Source: CAD feature listing. Evaluate the final solid. Frame: model axes, mm. A direction names the side the tool comes from. Coordinates: 2 decimals unless noted, no trailing zeros. Loops run counter-clockwise (first coordinate to the right, second up) from the corner with the lowest first, then second, coordinate; pieces in that order, holes last. Notation, with made-up numbers: (31.5, 72.5) - (66.5, 72.5) arc R19 ccw to (66.5, 94.5) - close; hole circle Ø4 at (66, -31). An arc over 180 degrees is marked (long way). Use CSV: the item, a comma, the result in double quotes. Start each with the question number.
```python
from build123d import *

# Parameters (mm, degrees)
FASE1_SIZE                      = 2
FASE2_SIZE                      = 4
FASE2_SIZE2                     = 1.377310453
FASE3_SIZE                      = 4
FASE3_SIZE2                     = 1.377310453
SCHNITT_LINEAR_AUSTRAGEN1_DEPTH = 9.5
FASE4_SIZE                      = 1
FASE4_SIZE2                     = 1.613032213
FASE5_SIZE                      = 1.623645291


with BuildPart() as part:
    # Skizze1 → Rotation1 (revolve)
    with BuildSketch(Plane.XY, mode=Mode.PRIVATE) as rotation1_sk:
        with BuildLine():
            Line((-2.51871264, 34.081541744), (-2.51871264, 15.53217569))
            Line((-2.51871264, 15.53217569), (-5.248906592, 12.857142857))
            ThreePointArc((-5.248906592, 12.857142857), (-7.478321416, 8.069832253), (-6, 3))
            Line((-6, 3), (-10, 3))
            Line((-10, 3), (-10, 15))
            Line((-10, 15), (-6, 15))
            Line((-6, 15), (-4.093652292, 16.867831662))
            Line((-4.093652292, 16.867831662), (-4.093652292, 20.696496392))
            ThreePointArc((-4.093652292, 20.696496392), (-7.464630082, 27.878319169), (-2.51871264, 34.081541744))
        make_face()
    revolve(rotation1_sk.sketch.rotate(Axis((0, 15, 0), (0, 1, 0)), 180), axis=Axis((0, 15, 0), (0, 1, 0)))

    # Fase1
    # the kernel refuses this chamfer: 2, 1.818354592 mm, written as the material it takes off along each edge
    with BuildSketch(Plane(origin=(0, 3, 0), x_dir=(1, 0, 0), z_dir=(0, 0, 1))) as fase1_piece_1:
        with BuildLine():
            Line((6.949872666, 1.680555032), (6 + FASE1_SIZE, 0))
            Line((6 + FASE1_SIZE, 0), (6, 0))
            ThreePointArc((6, 0), (6.538732617, 0.826449161), (6.949872666, 1.680555032))
        make_face()
    revolve(axis=Axis((0, 3, 0), (0, 1, 0)), mode=Mode.SUBTRACT)

    # Fase2
    fase2_edges = [part.edges().sort_by_distance(p)[0] for p in [
        (-10, 3, 0),
    ]]
    fase2_side = [part.faces().sort_by_distance(p)[0] for p in [
        (-10, 9, 0),
    ]]
    chamfer(fase2_edges, length=FASE2_SIZE, length2=FASE2_SIZE2, reference=fase2_side[0])

    # Fase3
    fase3_edges = [part.edges().sort_by_distance(p)[0] for p in [
        (-10, 15, 0),
    ]]
    fase3_side = [part.faces().sort_by_distance(p)[0] for p in [
        (-10, 11, 0),
    ]]
    chamfer(fase3_edges, length=FASE3_SIZE, length2=FASE3_SIZE2, reference=fase3_side[0])

    # Skizze2 → Schnitt-Linear austragen1 (cut)
    with BuildSketch(Plane.XZ.offset(-3)):
        Polygon((0, 10.698773164), (1, 10.698773164), (1, 1), (12.923434457, 1), (12.923434457, 0), (12.923434457, -1), (1, -1), (1, -10.815383619), (0, -10.815383619), (-1, -10.815383619), (-1, -1), (-10.582773881, -1), (-10.582773881, 0), (-10.582773881, 1), (-1, 1), (-1, 10.698773164), align=None)
    extrude(amount=-SCHNITT_LINEAR_AUSTRAGEN1_DEPTH, mode=Mode.SUBTRACT)

    # Fase4
    fase4_edges = [part.edges().sort_by_distance(p)[0] for p in [
        (-8.622689547, 15, 0),
    ]]
    fase4_side = [part.faces().sort_by_distance(p)[0] for p in [
        (-9.311344773, 13, 0),
    ]]
    chamfer(fase4_edges, length=FASE4_SIZE, length2=FASE4_SIZE2, reference=fase4_side[0])

    # Fase5
    # the kernel refuses this chamfer: 1.623645291, 1.5 mm, written as the material it takes off along each edge
    with BuildSketch(Plane(origin=(0, 34.081541744, 0), x_dir=(1, 0, 0), z_dir=(0, 0, 1))) as fase5_piece_1:
        with BuildLine():
            Line((2.51871264, -FASE5_SIZE), (3.807658871, -0.601273173))
            ThreePointArc((3.807658871, -0.601273173), (3.190605907, -0.276236403), (2.51871264, 0))
            Line((2.51871264, 0), (2.51871264, -FASE5_SIZE))
        make_face()
    revolve(axis=Axis((0, 34.081541744, 0), (0, 1, 0)), mode=Mode.SUBTRACT)


solid = part.part
```
(1) Draft query along Y for faces 1 (the conical face through (6.64, 4.97, -6.51)), 2 (the flat face through (1, 9, -8)), 3 (the cylindrical face through (-0.53, 18.81, -4.06)). Return one class per face: released by +Y, released by -Y, zero draft, split by the parting line, or undercut.
(2) Ray query, line 1 (Z direction, x = 0, y = 19.5); line 2 (X direction, y = 22.5, z = -0.75); line 3 (Y direction, x = -0.75, z = -6.5). Return the intervals inside material, ascending. Write a range as [from, to].
(3) Section C-C on y = 18. Output: boundary loops of the cut face in (x, z), plus the area to 3 significant figures.
(4) Pin query (flat end, axial travel): pin 1 Ø5 at (y, z) = (6.5, -8.5) entering from -X; pin 2 Ø10 at (y, z) = (29, 2.5) entering from -X; pin 3 Ø1.6 at (x, z) = (-8, 0) entering from -Y; pin 4 Ø3 at (x, z) = (0, 0) entering from -Y. Return the tip coordinate at first contact, or that it passes through.
(5) Section A-A on z = 0. Output: boundary loops of the cut face in (x, y).
(6) Reachability of faces 4 (the conical face through (-5.16, 4.015, -5.256)), 5 (the flat face through (8, 9, -1)), 6 (the flat face through (-1, 9, 8)), 7 (the flat face through (6, 15, -2)) from +Z, -Z, +X, -X, +Y, -Y: full face, straight path, thin tool, end or side. Return the list, or none.
(7) Section D-D on y = 23. Output: boundary loops of the cut face in (x, z), plus the area to 3 significant figures.
(8) Section B-B on x = 0. Output: boundary loops of the cut face in (y, z).
Solution:
1,face 1,"released by -Y"
1,face 2,"zero draft"
1,face 3,"undercut"
2,line 1,"z = [-4.09, -2.52], [2.52, 4.09]"
2,line 2,"x = [-5.97, -2.4], [2.4, 5.97]"
2,line 3,"y = [12.5, 15], [23.3, 30.7]"
3,outline,"circle Ø8.19 at (0, 0); hole circle Ø5.04 at (0, 0)"
3,area,"32.7 mm²"
4,pin 1,"stops at x = -7.96"
4,pin 2,"stops at x = -7.52"
4,pin 3,"stops at y = 12.5"
4,pin 4,"passes through"
5,outline,"(-9.48, 12.5) - (-5.59, 12.5) arc R7.5 cw to (-5.25, 12.86) - (-2.52, 15.53) - (-2.52, 32.46) - (-3.81, 33.48) arc R7.52 ccw to (-4.09, 20.7) - (-4.09, 16.87) - (-6, 15) - (-7.01, 15) - (-8.95, 14.05) - close; (2.52, 15.53) - (5.25, 12.86) arc R7.5 cw to (5.59, 12.5) - (9.48, 12.5) - (8.95, 14.05) - (7.01, 15) - (6, 15) - (4.09, 16.87) - (4.09, 20.7) arc R7.52 ccw to (3.81, 33.48) - (2.52, 32.46) - close"
6,face 4,"-Y"
6,face 5,"+X, -X, -Y"
6,face 6,"+Z, -Z, -Y"
6,face 7,"none"
7,outline,"circle Ø12.73 at (0, 0); hole circle Ø5.04 at (0, 0)"
7,area,"107 mm²"
8,outline,"(12.5, -9.48) - (14.05, -8.95) - (15, -7.01) - (15, -6) - (16.87, -4.09) - (20.7, -4.09) arc R7.52 ccw to (33.48, -3.81) - (32.46, -2.52) - (15.53, -2.52) - (12.86, -5.25) arc R7.5 cw to (12.5, -5.59) - close; (12.5, 5.59) arc R7.5 cw to (12.86, 5.25) - (15.53, 2.52) - (32.46, 2.52) - (33.48, 3.81) arc R7.52 ccw to (20.7, 4.09) - (16.87, 4.09) - (15, 6) - (15, 7.01) - (14.05, 8.95) - (12.5, 9.48) - close"
